Geometry: final body of the model. Coordinates: model frame, mm. Face numbers are marked on the shaded views. A direction names the side the tool comes from. Give positions to 0.01 mm unless a question says otherwise; leave off trailing zeros. Write each loop counter-clockwise with the first axis right and the second up, starting at its lowest first coordinate (ties: lowest second). Pieces come first, ordered by that corner, then holes.
Q1. Section B-B (y = -58). Return the cut outline in (x, z).
Q2. Section A-A (z = -6.5). Return the cut outline in (x, y).
Q3. Line query: line 1 (Z direction, x = 55, y = -66); line 2 (Y direction, x = 4.5, z = -12.5); line 3 (X direction, y = -35, z = 22). Output: solid intervals per line, ascending.
Q4. Pin query (flat end, axial travel): pin 1 Ø5 at (y, z) = (-34.5, 26) entering from -X; pin 2 Ø8 at (x, z) = (23.5, -7) entering from +Y; pin 3 Ø6 at (y, z) = (9.5, 14.5) entering from -X; pin 4 Ø24 at (x, y) = (57.99, -37.89) entering from +Z. Return the tip coordinate at first contact, or that it passes through.
Q5. Mould query, pull axis X, two halves, no side actions, for the marked faces 3, 4 and 5. Classes: +X half, -X half, draft (parallel to the pull), parting line (faces both ways), or undercut.
Q6. Reachability of the marked faces 1 and 2 from +Z, -Z, +X, -X, +Y, -Y: full face, straight path, thin tool, end or side. Return the list, or none.
Q7. Section C-C (x = 45). State how many separate pieces and enclosed holes the cut face has, plus the area to 3 significant figures.
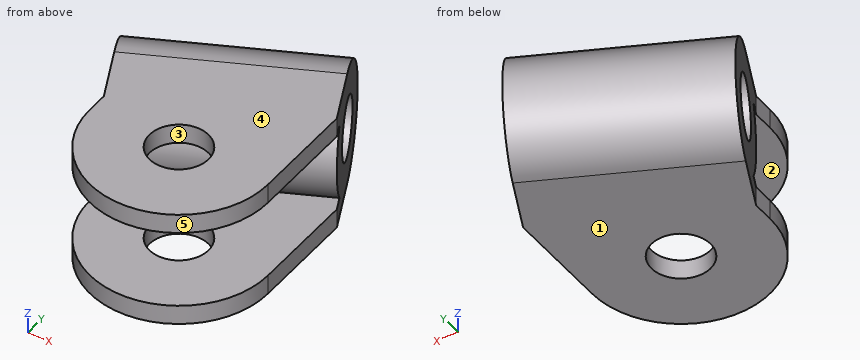
from build123d import *

# Parameters (mm, degrees)
BOSS_EXTRUDE1_START     = 20
BOSS_EXTRUDE1_DEPTH     = 10
BOSS_EXTRUDE2_START     = -20
BOSS_EXTRUDE2_DEPTH     = 10
SKETCH3_W               = 100
SKETCH3_H               = 10
BOSS_EXTRUDE3_DEPTH     = 30
SKETCH4_R               = 15
CUT_EXTRUDE1_DEPTH      = 23.981333294
CUT_EXTRUDE1_DEPTH_BACK = 147.654073313
SKETCH5_R               = 15
CUT_EXTRUDE2_DEPTH      = 1
CUT_EXTRUDE2_DEPTH_BACK = 61


with BuildPart() as part:
    # Sketch1 → Revolve1 (revolve)
    with BuildSketch(Plane.XY):
        Polygon((0, 0), (90.630778704, 42.261826174), (77.952230851, 69.451059785), (-12.678547852, 27.189233611), align=None)
    revolve(axis=Axis((0, 0, 0), (0.906307787, 0.422618262, 0)))



with BuildPart() as body_2:
    # Sketch2 → Boss-Extrude1 (new body)
    with BuildSketch(Plane.XY.offset(BOSS_EXTRUDE1_START)):
        with BuildLine():
            Line((12.678547852, -27.189233611), (12.678547852, -37.88831917))
            ThreePointArc((12.678547852, -37.88831917), (57.993937204, -83.203708522), (103.309326556, -37.88831917))
            Line((103.309326556, -37.88831917), (103.309326556, 15.072592563))
            Line((103.309326556, 15.072592563), (12.678547852, -27.189233611))
        make_face()
    extrude(amount=BOSS_EXTRUDE1_DEPTH)


with BuildPart() as body_3:
    # Sketch2<3> → Boss-Extrude2 (new body)
    with BuildSketch(Plane.XY.offset(BOSS_EXTRUDE2_START)):
        with BuildLine():
            Line((12.678547852, -27.189233611), (12.678547852, -37.88831917))
            ThreePointArc((12.678547852, -37.88831917), (57.993937204, -83.203708522), (103.309326556, -37.88831917))
            Line((103.309326556, -37.88831917), (103.309326556, 15.072592563))
            Line((103.309326556, 15.072592563), (12.678547852, -27.189233611))
        make_face()
    extrude(amount=-BOSS_EXTRUDE2_DEPTH)


with BuildPart() as part_1:
    add(part.part)

    add(body_2.part)  # Boss-Extrude3 merges body 2

    add(body_3.part)  # Boss-Extrude3 merges body 3
    # Sketch3 → Boss-Extrude3 (add)
    with BuildSketch(Plane(origin=(12.678547852, -27.189233611, 0), x_dir=(0.906307787, 0.422618262, 0), z_dir=(-0.422618262, 0.906307787, 0))):
        with Locations((50, -25)):
            Rectangle(SKETCH3_W, SKETCH3_H)
        with Locations((50, 25)):
            Rectangle(SKETCH3_W, SKETCH3_H)
    extrude(amount=BOSS_EXTRUDE3_DEPTH)

    # Sketch4 → Cut-Extrude1 (cut, two sides)
    with BuildSketch(Plane(origin=(90.630778704, 42.261826174, 0), x_dir=(0, 0, -1), z_dir=(0.906307787, 0.422618262, 0))) as cut_extrude1_sk:
        Circle(SKETCH4_R)
    extrude(amount=CUT_EXTRUDE1_DEPTH, mode=Mode.SUBTRACT)
    extrude(cut_extrude1_sk.sketch, amount=-CUT_EXTRUDE1_DEPTH_BACK, mode=Mode.SUBTRACT)

    # Sketch5 → Cut-Extrude2 (cut, two sides)
    with BuildSketch(Plane.XY.offset(30)) as cut_extrude2_sk:
        with Locations((57.993937204, -37.88831917)):
            Circle(SKETCH5_R)
    extrude(amount=CUT_EXTRUDE2_DEPTH, mode=Mode.SUBTRACT)
    extrude(cut_extrude2_sk.sketch, amount=-CUT_EXTRUDE2_DEPTH_BACK, mode=Mode.SUBTRACT)


solid = part_1.part
Computed:
1. outline: (17.39, -30) - (98.6, -30) - (98.6, -20) - (17.39, -20) - close; (17.39, 20) - (98.6, 20) - (98.6, 30) - (17.39, 30) - close
2. outline: (-12.38, 26.54) - (-5.71, 12.25) - (84.92, 54.51) - (78.25, 68.81) - close; (5.71, -12.25) - (12.38, -26.54) - (103.01, 15.72) - (96.34, 30.01) - close
3. line 1: z = -30 to -20, 20 to 30
3. line 2: y = -9.65 to -7.05, 11.25 to 32.19
3. line 3: x = 12.68 to 43.27, 72.71 to 103.31
4. pin 1: stops at x = 12.68
4. pin 2: stops at y = 45.23
4. pin 3: stops at x = -5.83
4. pin 4: passes through
5. face 3: undercut
5. face 4: draft
5. face 5: parting line
6. face 1: -Z, +X, -X, +Y, -Y
6. face 2: +X, -Y
7. separate pieces: 3
7. enclosed holes: 1
7. area: 3,740 mm2
